from build123d import *

# Parameters (mm, degrees)
ESQUISSE1_W        = 680
ESQUISSE1_H        = 90
ESQUISSE1_R        = 2.75
ESQUISSE1_R_2      = 2.25
ESQUISSE1_R_3      = 4
BOSS_EXTRU_1_DEPTH = 8
ESQUISSE2_W        = 8
ESQUISSE2_H        = 90
BOSS_EXTRU_2_DEPTH = 20
ESQUISSE3_W        = 8
ESQUISSE3_H        = 90
BOSS_EXTRU_3_DEPTH = 20


with BuildPart() as part:
    # Esquisse1 → Boss.-Extru.1 (new body)
    with BuildSketch(Plane.XY):
        with Locations((340, 45)):
            Rectangle(ESQUISSE1_W, ESQUISSE1_H)
        with Locations((317, 48.92)):
            Circle(ESQUISSE1_R, mode=Mode.SUBTRACT)
        with Locations((363, 48.92)):
            Circle(ESQUISSE1_R, mode=Mode.SUBTRACT)
        with Locations((316.45, 72.47)):
            Circle(ESQUISSE1_R_2, mode=Mode.SUBTRACT)
        with Locations((363.55, 72.47)):
            Circle(ESQUISSE1_R_2, mode=Mode.SUBTRACT)
        with Locations(Location((363.55, 25.37, 0), (0, 0, 180))):
            Circle(ESQUISSE1_R_2, mode=Mode.SUBTRACT)
        with Locations(Location((316.45, 25.37, 0), (0, 0, 180))):
            Circle(ESQUISSE1_R_2, mode=Mode.SUBTRACT)
        with Locations((35.3, 75)):
            Circle(ESQUISSE1_R_3, mode=Mode.SUBTRACT)
        with Locations((35.3, 45)):
            Circle(ESQUISSE1_R_3, mode=Mode.SUBTRACT)
        with Locations(Location((644.7, 45, 0), (0, 0, 180))):
            Circle(ESQUISSE1_R_3, mode=Mode.SUBTRACT)
        with Locations(Location((644.7, 75, 0), (0, 0, 180))):
            Circle(ESQUISSE1_R_3, mode=Mode.SUBTRACT)
        with Locations((155.3, 75)):
            Circle(ESQUISSE1_R_3, mode=Mode.SUBTRACT)
        with Locations((155.3, 45)):
            Circle(ESQUISSE1_R_3, mode=Mode.SUBTRACT)
        with Locations((275.3, 75)):
            Circle(ESQUISSE1_R_3, mode=Mode.SUBTRACT)
        with Locations((275.3, 45)):
            Circle(ESQUISSE1_R_3, mode=Mode.SUBTRACT)
        with Locations(Location((404.7, 45, 0), (0, 0, 180))):
            Circle(ESQUISSE1_R_3, mode=Mode.SUBTRACT)
        with Locations(Location((404.7, 75, 0), (0, 0, 180))):
            Circle(ESQUISSE1_R_3, mode=Mode.SUBTRACT)
        with Locations(Location((524.7, 75, 0), (0, 0, 180))):
            Circle(ESQUISSE1_R_3, mode=Mode.SUBTRACT)
        with Locations(Location((524.7, 45, 0), (0, 0, 180))):
            Circle(ESQUISSE1_R_3, mode=Mode.SUBTRACT)
        with BuildLine():
            Line((340, 30.92), (355, 30.92))
            ThreePointArc((355, 30.92), (357.121320344, 31.798679656), (358, 33.92))
            Line((358, 33.92), (358, 63.92))
            ThreePointArc((358, 63.92), (357.121320344, 66.041320344), (355, 66.92))
            Line((355, 66.92), (325, 66.92))
            ThreePointArc((325, 66.92), (322.878679656, 66.041320344), (322, 63.92))
            Line((322, 63.92), (322, 33.92))
            ThreePointArc((322, 33.92), (322.878679656, 31.798679656), (325, 30.92))
            Line((325, 30.92), (340, 30.92))
        make_face(mode=Mode.SUBTRACT)
    extrude(amount=BOSS_EXTRU_1_DEPTH)

    # Esquisse2 → Boss.-Extru.2 (add)
    with BuildSketch(Plane(origin=(680, 0, 0), x_dir=(0, 0, -1), z_dir=(1, 0, 0))):
        with Locations((-4, 45)):
            Rectangle(ESQUISSE2_W, ESQUISSE2_H)
    extrude(amount=BOSS_EXTRU_2_DEPTH)

    # Esquisse3 → Boss.-Extru.3 (add)
    with BuildSketch(Plane.ZY):
        with Locations((4, 45)):
            Rectangle(ESQUISSE3_W, ESQUISSE3_H)
    extrude(amount=BOSS_EXTRU_3_DEPTH)


solid = part.part
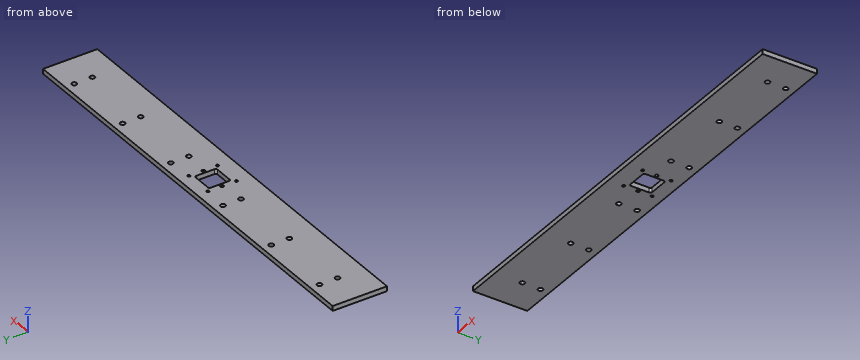
Read the model definition and answer for the solid it produces. Units are mm, in the model's axes. Round coordinates to 2 decimals unless told otherwise and drop trailing zeros.
Q1. Each of these flat-tipped pins is pushed along its axis until it touches: pin 1 (13 mm diameter, centred on x = 524.7, y = 45, fed in from +Z); pin 2 (2.5 mm diameter, centred on x = 316.45, y = 72.47, fed in from -Z). Where does it stop, or does it pass through?
Q2. Section A-A on z = 1.25 is taken. Give the number of separate pieces and of enclosed holes in the cut face, and give its area (3 significant figures).
Q3. Consider probe 1 along Y at (x, z) = (155.3, 3); probe 2 along Y at (x, z) = (317, 6); probe 3 along X at (y, z) = (25.37, 4.5). Determine where each line is inside the solid, lowest interval first.
Output:
1. pin 1: stops at z = 8
1. pin 2: passes through
2. separate pieces: 1
2. enclosed holes: 19
2. area: 62,800 mm2
3. probe 1: y = 0 to 41, 49 to 71, 79 to 90
3. probe 2: y = 0 to 23.19, 27.55 to 46.17, 51.67 to 70.29, 74.65 to 90
3. probe 3: x = -20 to 314.2, 318.7 to 361.3, 365.8 to 700
